Could you check a few things on this model? Use its own coordinates, in mm. A direction names the side the tool comes from. Coordinates: 2 decimals unless noted, no trailing zeros.
from build123d import *

# Parameters (mm, degrees)
SKETCH2_W               = 75
SKETCH2_H               = 45
BOSS_EXTRUDE1_DEPTH     = 20
SKETCH3_W               = 110
SKETCH3_H               = 80
BOSS_EXTRUDE2_DEPTH     = 10
SKETCH4_W               = 1.25
SKETCH4_H               = 2.8
CUT_EXTRUDE1_DEPTH      = 10
SKETCH5_W               = 30
SKETCH5_H               = 80
BOSS_EXTRUDE4_DEPTH     = 10
SKETCH8_R               = 1.5
CUT_EXTRUDE2_DEPTH      = 120
SKETCH9_R               = 2.5
CUT_EXTRUDE3_DEPTH      = 40
CUT_EXTRUDE3_DEPTH_BACK = 20
SKETCH10_W              = 3.7
SKETCH10_H              = 8
CUT_EXTRUDE4_DEPTH      = 15
FILLET1_R               = 2.5


with BuildPart() as part:
    # Sketch2 → Boss-Extrude1 (new body)
    with BuildSketch(Plane.XY):
        Polygon((42.5, -22.5), (42.5, 22.5), (55, 22.5), (55, 40), (-55, 40), (-55, -40), (55, -40), (55, -22.5), align=None)
        with BuildLine():
            Line((-37.5, -22.5), (-37.5, 22.5))
            Line((-37.5, 22.5), (-37.5, 26))
            ThreePointArc((-37.5, 26), (-40.328427125, 32.828427125), (-33.5, 30))
            Line((-33.5, 30), (33.5, 30))
            ThreePointArc((33.5, 30), (37.5, 34), (41.5, 30))
            ThreePointArc((41.5, 30), (40.328427125, 27.171572875), (37.5, 26))
            Line((37.5, 26), (37.5, 22.5))
            Line((37.5, 22.5), (37.5, -22.5))
            Line((37.5, -22.5), (37.5, -26))
            ThreePointArc((37.5, -26), (40.328427125, -27.171572875), (41.5, -30))
            ThreePointArc((41.5, -30), (37.5, -34), (33.5, -30))
            Line((33.5, -30), (-33.5, -30))
            ThreePointArc((-33.5, -30), (-40.328427125, -32.828427125), (-37.5, -26))
            Line((-37.5, -26), (-37.5, -22.5))
        make_face(mode=Mode.SUBTRACT)
        with BuildLine():
            Line((-37.5, 26), (-37.5, 22.5))
            Line((-37.5, 22.5), (37.5, 22.5))
            Line((37.5, 22.5), (37.5, 26))
            ThreePointArc((37.5, 26), (34.671572875, 27.171572875), (33.5, 30))
            Line((33.5, 30), (-33.5, 30))
            ThreePointArc((-33.5, 30), (-34.671572875, 27.171572875), (-37.5, 26))
        make_face()
        Rectangle(SKETCH2_W, SKETCH2_H)
        with BuildLine():
            Line((37.5, -22.5), (-37.5, -22.5))
            Line((-37.5, -22.5), (-37.5, -26))
            ThreePointArc((-37.5, -26), (-34.671572875, -27.171572875), (-33.5, -30))
            Line((-33.5, -30), (33.5, -30))
            ThreePointArc((33.5, -30), (34.671572875, -27.171572875), (37.5, -26))
            Line((37.5, -26), (37.5, -22.5))
        make_face()
    extrude(amount=BOSS_EXTRUDE1_DEPTH)

    # Sketch3 → Boss-Extrude2 (add)
    with BuildSketch(Plane.XY.offset(20)):
        Rectangle(SKETCH3_W, SKETCH3_H)
    extrude(amount=BOSS_EXTRUDE2_DEPTH)

    # Sketch4 → Cut-Extrude1 (cut)
    with BuildSketch(Plane.XY):
        Polygon((43.75, 32.8), (43.75, 30), (45, 30), (45, 27.2), (46.25, 27.2), (46.25, 32.8), align=None)
        with Locations((44.375, 28.6)):
            Rectangle(SKETCH4_W, SKETCH4_H)
        Polygon((-45, 27.2), (-45, 30), (-43.75, 30), (-43.75, 32.8), (-46.25, 32.8), (-46.25, 27.2), align=None)
        with Locations((-44.375, 28.6)):
            Rectangle(SKETCH4_W, SKETCH4_H)
        with Locations((-44.375, -28.6)):
            Rectangle(SKETCH4_W, SKETCH4_H)
        Polygon((-45, -30), (-45, -27.2), (-46.25, -27.2), (-46.25, -32.8), (-43.75, -32.8), (-43.75, -30), align=None)
        Polygon((46.25, -27.2), (45, -27.2), (45, -30), (43.75, -30), (43.75, -32.8), (46.25, -32.8), align=None)
        with Locations((44.375, -28.6)):
            Rectangle(SKETCH4_W, SKETCH4_H)
    extrude(amount=CUT_EXTRUDE1_DEPTH, mode=Mode.SUBTRACT)

    # Sketch5 → Boss-Extrude4 (add)
    with BuildSketch(Plane(origin=(55, 0, 0), x_dir=(0, 0, -1), z_dir=(1, 0, 0))):
        with Locations((-15, 0)):
            Rectangle(SKETCH5_W, SKETCH5_H)
    extrude(amount=BOSS_EXTRUDE4_DEPTH)

    # Sketch8 → Cut-Extrude2 (cut)
    with BuildSketch(Plane(origin=(65, 0, 0), x_dir=(0, 0, -1), z_dir=(1, 0, 0))):
        with Locations((-6.5, 30)):
            Circle(SKETCH8_R)
        with Locations((-6.5, -30)):
            Circle(SKETCH8_R)
    extrude(amount=-CUT_EXTRUDE2_DEPTH, mode=Mode.SUBTRACT)

    # Sketch9 → Cut-Extrude3 (cut, two sides)
    with BuildSketch(Plane(origin=(42.5, 0, 0), x_dir=(0, 0, -1), z_dir=(1, 0, 0))) as cut_extrude3_sk:
        with Locations((-10, 0)):
            Circle(SKETCH9_R)
    extrude(amount=CUT_EXTRUDE3_DEPTH, mode=Mode.SUBTRACT)
    extrude(cut_extrude3_sk.sketch, amount=-CUT_EXTRUDE3_DEPTH_BACK, mode=Mode.SUBTRACT)

    # Sketch10 → Cut-Extrude4 (cut)
    with BuildSketch(Plane(origin=(0, 0, 0), x_dir=(-1, 0, 0), z_dir=(0, 0, -1))):
        with Locations((-35.65, 0)):
            Rectangle(SKETCH10_W, SKETCH10_H)
        with Locations((-59.35, 0)):
            Rectangle(SKETCH10_W, SKETCH10_H)
    extrude(amount=-CUT_EXTRUDE4_DEPTH, mode=Mode.SUBTRACT)

    # Fillet1
    fillet1_edges = [part.edges().sort_by_distance(p)[0] for p in [
        (65, -40, 15),
        (65, 40, 15),
        (-55, -40, 15),
        (-55, 40, 15),
    ]]
    fillet(fillet1_edges, radius=FILLET1_R)


solid = part.part
(1) For pin 1 (0.8 mm diameter, centred on x = 45.5, y = -30, fed in from -Z); pin 2 (1.8 mm diameter, centred on y = 30, z = 6.5, fed in from -X); pin 3 (5 mm diameter, centred on x = -37.5, y = 30, fed in from -Z), each with a flat end and sliding along its axis, tell me the tip position at first contact or that it passes through.
Answers:
pin 1: stops at z = 10
pin 2: passes through
pin 3: stops at z = 20
(2) We'd pull the mould along Y, two halves only. Please class faces 1 (the face through (-45, 32.8, 5)), 2 (the face through (64.287, 39.248, 14.79)), 3 (the face through (-54.287, -39.248, 15.21)), 4 (the face through (0.473, -30.575, 5.114)): +Y half, -Y half, draft (parallel to the pull), parting line (faces both ways), or undercut.
Answers:
face 1: undercut
face 2: +Y half
face 3: -Y half
face 4: undercut
(3) Imagine slicing it at A-A, the plane y = 0. State how many separate pieces and enclosed holes the cut face has, and give its area (3 significant figures).
Answers:
separate pieces: 4
enclosed holes: 0
area: 3,130 mm2
(4) Which directions (+Z, -Z, +X, -X, +Y, -Y) give clear straight access to the entire face, cutting with the end or side of a thin tool? Please do faces 5 (the face through (-42, -30, 5)), 6 (the face through (40, 0.1, 12.5)), 7 (the face through (49, 0, 20)).
Answers:
face 5: +X, -X
face 6: +X
face 7: -Z
(5) I need wall thicknesses on probe 1 along X at (y, z) = (31.5, 14); probe 2 along Y at (x, z) = (62.15, 10); probe 3 along Y at (x, z) = (-52.25, 6.5). Which ranges of each line are inside material? Lowest first, please.
Answers:
probe 1: x = -55 to -41.21, -33.79 to 33.79, 41.21 to 65
probe 2: y = -40 to -2.5, 2.5 to 40
probe 3: y = -40 to -31.5, -28.5 to 28.5, 31.5 to 40
